Study the drawing (mm; zero at the part's minimum x, y, z) and answer. A direction names the side the tool comes from. Coordinates: 2 decimals unless noted, no trailing zeros. Order: outer loops, then holes, each group sorted by start corner. A loop starts at its lowest first (then second) coordinate and runs counter-clockwise, first axis right, second up. Notation, with made-up numbers: (-35.75, 5) -> (-12.75, 5) arc R12 ccw to (-12.75, 22) -> close; hole circle Ø10 at (37, 40.25). An arc over 180 degrees is marked (long way). Answer as CSV lines item,"result". Start each with the question number.
Item 1: For a pull along Y with two mould halves and no side action, classify the marked faces 4, 5 and 6 as pulls with the +Y half, pulls with the -Y half, needs draft (parallel to the pull), parting line crosses it, or undercut.
Item 2: Which of the six approach directions +Z, -Z, +X, -X, +Y, -Y give full straight-line access (tool end or side, diameter ignored) to the marked faces 1, 2 and 3?
Item 3: Each of these flat-tipped pins is pushed along its axis until it touches: pin 1 Ø8 at (x, z) = (6, 11) entering from +Y; pin 2 Ø2.5 at (x, y) = (12.5, 22) entering from +Z; pin 3 Ø4 at (x, z) = (7, 9.5) entering from -Y; pin 4 Ø1 at (y, z) = (11.5, 13.5) entering from +X. Where does it stop, or does it pass through?
Item 4: Section D-D (z = 10.5) is taken. Write down the section's boundary in (x, y).
Item 5: Straight lines are drawn through the part: L1, parallel to Y at x = 12.5, z = 9.6; L2, parallel to Y at x = 12.5, z = 12.15; L3, parallel to Z at x = 6, y = 17.75. For each, find the intervals that lie inside material, in ascending order.
Item 6: Section A-A (y = 12.5) is taken. Write down the section's boundary in (x, z).
Item 7: Section C-C (y = 3) is taken. Write down the section's boundary in (x, z), then the cut area to 3 significant figures.
Item 8: Section B-B (x = 8.5) is taken. Write down the section's boundary in (y, z).
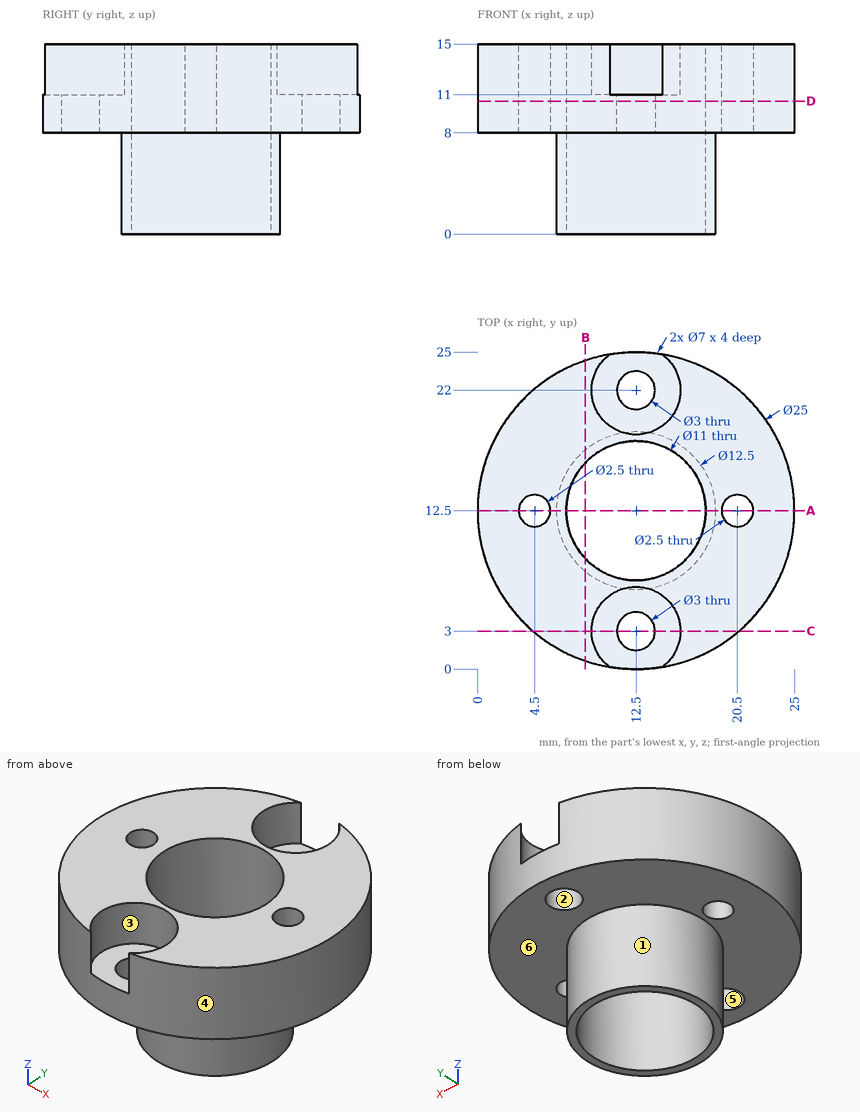
Checked values:
1,face 4,"parting line crosses it"
1,face 5,"undercut"
1,face 6,"needs draft"
2,face 1,"-Z"
2,face 2,"+Z, -Z"
2,face 3,"+Z"
3,pin 1,"stops at y = 24.75"
3,pin 2,"passes through"
3,pin 3,"stops at y = 0.5"
3,pin 4,"stops at x = 24.99"
4,outline,"circle Ø25 at (12.5, 12.5); hole circle Ø2.5 at (4.5, 12.5); hole circle Ø11 at (12.5, 12.5); hole circle Ø3 at (12.5, 3); hole circle Ø3 at (12.5, 22); hole circle Ø2.5 at (20.5, 12.5)"
5,L1,"y = 0 to 1.5, 4.5 to 7, 18 to 20.5, 23.5 to 25"
5,L2,"y = 6.5 to 7, 18 to 18.5"
5,L3,"z = 8 to 15"
6,outline,"(0, 8) -> (3.25, 8) -> (3.25, 15) -> (0, 15) -> close; (5.75, 8) -> (6.25, 8) -> (6.25, 0) -> (7, 0) -> (7, 15) -> (5.75, 15) -> close; (18, 0) -> (18.75, 0) -> (18.75, 8) -> (19.25, 8) -> (19.25, 15) -> (18, 15) -> close; (21.75, 8) -> (25, 8) -> (25, 15) -> (21.75, 15) -> close"
7,outline,"(4.38, 8) -> (11, 8) -> (11, 11) -> (9, 11) -> (9, 15) -> (4.38, 15) -> close; (14, 8) -> (20.62, 8) -> (20.62, 15) -> (16, 15) -> (16, 11) -> (14, 11) -> close"
7,area,"76.7 mm^2"
8,outline,"(0.66, 8) -> (7.7, 8) -> (7.7, 0) -> (8.73, 0) -> (8.73, 15) -> (0.66, 15) -> close; (16.27, 0) -> (17.3, 0) -> (17.3, 8) -> (24.34, 8) -> (24.34, 15) -> (16.27, 15) -> close"
